The figure shows three views and two pictorial views of one solid part (mm, origin at its lowest corner). Answer the questions. A direction names the side the tool comes from. Coordinates: 2 decimals unless noted, no trailing zeros. Write each loop counter-clockwise with the first axis right and the second up, starting at its lowest first coordinate (ties: lowest second). Pieces come first, ordered by that corner, then holes. Notation, with made-up numbers: M 18,68.5 L 49,68.5 A14 ccw 49,73.5 Z; hole C -12,78 d8. An arc over 180 degrees is marked long. Use CSV: the item, a comma, the result in double quotes.
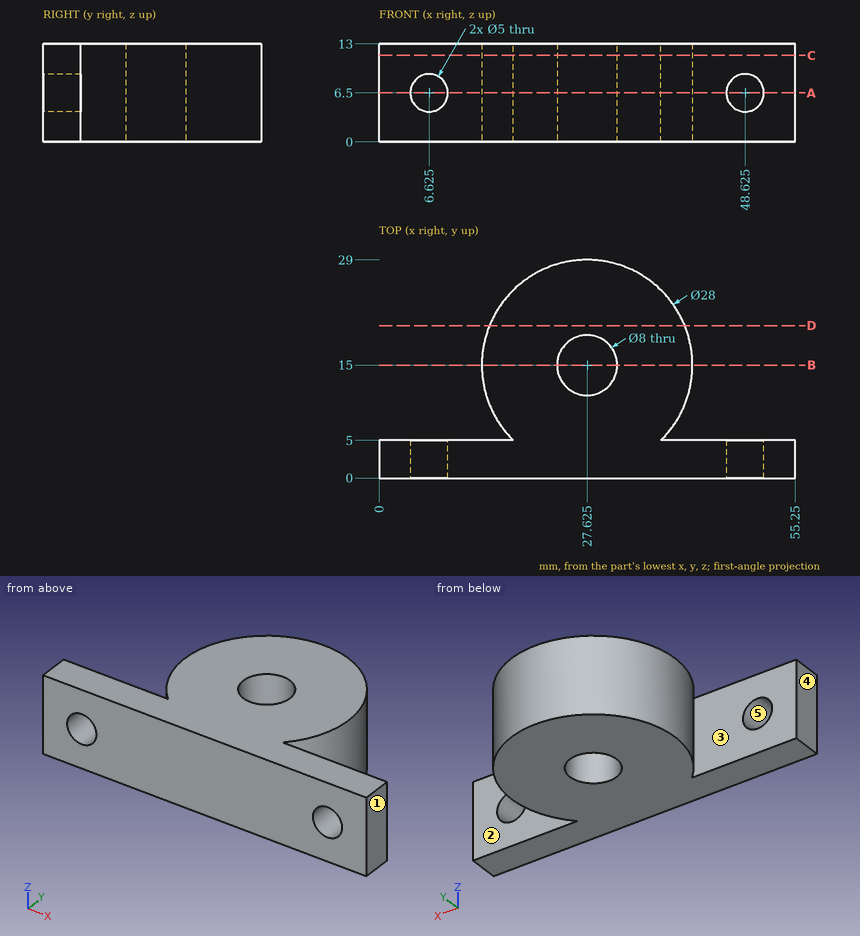
Item 1: The part is cut by section B-B (y = 15). Write down the section's boundary in (x, z) (3 decimals), then the cut area to 3 significant figures.
Answer:
outline,"M 13.625,0 L 23.625,0 L 23.625,13 L 13.625,13 Z; M 31.625,0 L 41.625,0 L 41.625,13 L 31.625,13 Z"
area,"260 mm2"
Item 2: Consider probe 1 along Y at (x, z) = (27.5, 1.5); probe 2 along X at (y, z) = (18.5, 2.25); probe 3 along Y at (x, z) = (12.5, 11). Determine where each line is inside the solid, lowest interval first.
Answer:
probe 1,"y = 0 to 11, 19 to 29"
probe 2,"x = 14.07 to 25.69, 29.56 to 41.18"
probe 3,"y = 0 to 5"
Item 3: The part is cut by section D-D (y = 20.25). Write down the section's boundary in (x, z).
Answer:
outline,"M 14.65,0 L 40.6,0 L 40.6,13 L 14.65,13 Z"
Item 4: The part is cut by section A-A (z = 6.5). Write down the section's boundary in (x, y) (3 decimals).
Answer:
outline,"M 0,0 L 4.125,0 L 4.125,5 L 0,5 Z; M 9.125,0 L 46.125,0 L 46.125,5 L 37.423,5 A14 ccw long 17.827,5 L 9.125,5 Z; M 51.125,0 L 55.25,0 L 55.25,5 L 51.125,5 Z; hole C 27.625,15 d8"
Item 5: For a pull along X with two mould halves and no side action, classify the marked faces 3, 4 and 5 as released by +X, released by -X, zero draft, split by the parting line, or undercut.
Answer:
face 3,"zero draft"
face 4,"released by -X"
face 5,"undercut"
Item 6: A tool of negligible diameter and unlimited length cuts with its end or side. For the marked faces 1 and 2, from which of +Z, -Z, +X, -X, +Y, -Y can it reach the whole face along a straight path? Write none if from no direction.
Answer:
face 1,"+Z, -Z, +X, +Y, -Y"
face 2,"+Z, -Z, +X"
Item 7: Given pin 1 (1.5 mm diameter, centred on y = 25.5, z = 8.5, fed in from +X); pin 2 (6 mm diameter, centred on x = 6.625, z = 6.5, fed in from +Y); pin 3 (7 mm diameter, centred on x = 27.625, y = 15, fed in from -Z); pin 4 (3 mm diameter, centred on y = 11, z = 8, fed in from +X), each flat-ended and moving along its own axis, determine where each tip first touches the part or whether it passes through.
Answer:
pin 1,"stops at x = 37.67"
pin 2,"stops at y = 5"
pin 3,"passes through"
pin 4,"stops at x = 41.4"
Item 8: The part is cut by section C-C (z = 11.5). Write down the section's boundary in (x, y) (3 decimals), then the cut area to 3 significant figures.
Answer:
outline,"M 0,0 L 55.25,0 L 55.25,5 L 37.423,5 A14 ccw long 17.827,5 L 0,5 Z; hole C 27.625,15 d8"
area,"788 mm2"
